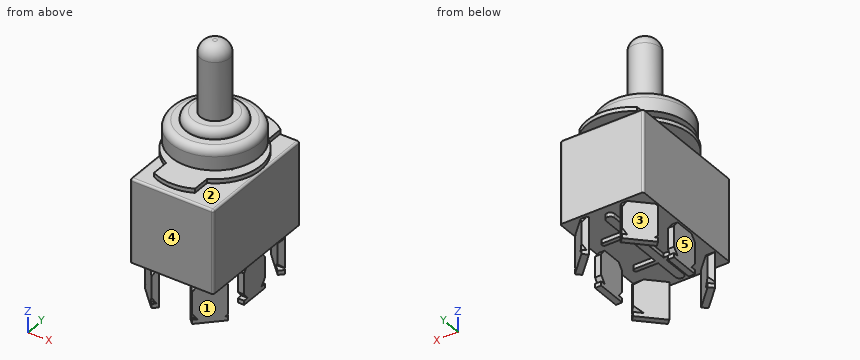
```python
from build123d import *

# Parameters (mm, degrees)
SKETCH_W     = 20
SKETCH_H     = 30
PAD_DEPTH    = 20
PAD001_DEPTH = 1.75
PAD002_DEPTH = 1
PAD003_DEPTH = 1.75
SKETCH004_R  = 10.5
PAD004_DEPTH = 5
SKETCH005_R  = 7
PAD005_DEPTH = 2
SKETCH006_R  = 3.5
PAD006_DEPTH = 17
FILLET_R     = 3
FILLET001_R  = 0.5
FILLET002_R  = 1.75
SKETCH007_W  = 1.5
SKETCH007_H  = 7.25
PAD007_DEPTH = 9
POCKET_DEPTH = 21.001
PAD008_DEPTH = 1


with BuildPart() as part:
    # Sketch → Pad (new body)
    with BuildSketch(Plane.XY):
        Rectangle(SKETCH_W, SKETCH_H)
    extrude(amount=PAD_DEPTH)

    # Sketch001 (on Face6 of Pad) → Pad001 (join)
    with BuildSketch(Plane.XY.offset(20)):
        Polygon((0, -8.313844), (7.2, -4.156922), (7.2, 4.156922), (0, 8.313844), (-7.2, 4.156922), (-7.2, -4.156922), align=None)
    extrude(amount=PAD001_DEPTH)

    # Sketch002 (on Face13 of Pad001) → Pad002 (join)
    with BuildSketch(Plane.XY.offset(21.75)):
        with BuildLine():
            ThreePointArc((6.924821, 12.746745), (0, 15.2), (-6.924821, 12.746745))
            Line((-6.924821, 8.546745), (-6.924821, 12.746745))
            ThreePointArc((-6.924821, 8.546745), (-10.934933, -1.194675), (-4.915971, -9.840388))
            Line((-4.915971, -9.840388), (-4.915971, -14.040388))
            ThreePointArc((-4.915971, -14.040388), (0, -15.2), (4.915971, -14.040388))
            Line((4.915971, -14.040388), (4.915971, -9.840388))
            ThreePointArc((4.915971, -9.840388), (10.934933, -1.194675), (6.924821, 8.546745))
            Line((6.924821, 12.746745), (6.924821, 8.546745))
        make_face()
    extrude(amount=PAD002_DEPTH)

    # Sketch003 (on Face22 of Pad002) → Pad003 (join)
    with BuildSketch(Plane.XY.offset(22.75)):
        Polygon((7.2, 4.156922), (0, 8.313844), (-7.2, 4.156922), (-7.2, -4.156922), (0, -8.313844), (7.2, -4.156922), align=None)
    extrude(amount=PAD003_DEPTH)

    # Sketch004 (on Face29 of Pad003) → Pad004 (join)
    with BuildSketch(Plane.XY.offset(24.5)):
        Circle(SKETCH004_R)
    extrude(amount=PAD004_DEPTH)

    # Sketch005 (on Face31 of Pad004) → Pad005 (join)
    with BuildSketch(Plane.XY.offset(29.5)):
        Circle(SKETCH005_R)
    extrude(amount=PAD005_DEPTH)

    # Sketch006 (on Face33 of Pad005) → Pad006 (join)
    with BuildSketch(Plane.XY.offset(31.5)):
        Circle(SKETCH006_R)
    extrude(amount=PAD006_DEPTH)

    # Fillet
    fillet_edges = [part.edges().sort_by_distance(p)[0] for p in [
        (-3.5, 0, 48.5),
    ]]
    fillet(fillet_edges, radius=FILLET_R)

    # Fillet001
    fillet001_edges = [part.edges().sort_by_distance(p)[0] for p in [
        (10, 15, 10),
        (10, -15, 10),
        (-10, -15, 10),
        (-10, 15, 10),
        (-10, 0, 20),
        (0, -15, 20),
        (10, 0, 20),
        (0, 15, 20),
    ]]
    fillet(fillet001_edges, radius=FILLET001_R)

    # Fillet002
    fillet002_edges = [part.edges().sort_by_distance(p)[0] for p in [
        (-10.5, 0, 29.5),
        (-7, 0, 31.5),
    ]]
    fillet(fillet002_edges, radius=FILLET002_R)

    # Sketch007 (on Face47 of Fillet002) → Pad007 (join)
    with BuildSketch(Plane(origin=(0, 0, 0), x_dir=(1, 0, 0), z_dir=(0, 0, -1))):
        Polygon((4.873476, 15), (10, 9.873476), (8.93934, 8.812816), (3.812816, 13.93934), align=None)
        with Locations((8.75, 0)):
            Rectangle(SKETCH007_W, SKETCH007_H)
        Polygon((-4.873476, 15), (-10, 9.873476), (-8.93934, 8.812816), (-3.812816, 13.93934), align=None)
        with Locations((-8.75, 0)):
            Rectangle(SKETCH007_W, SKETCH007_H)
        Polygon((4.873476, -15), (10, -9.873476), (8.93934, -8.812816), (3.812816, -13.93934), align=None)
        Polygon((-4.873476, -15), (-10, -9.873476), (-8.93934, -8.812816), (-3.812816, -13.93934), align=None)
    extrude(amount=PAD007_DEPTH)

    # Sketch008 (on Face39 of Pad007) → Pocket (cut, through all)
    with BuildSketch(Plane(origin=(-10, 0, 0), x_dir=(0, -1, 0), z_dir=(-1, 0, 0))):
        Polygon((-15, 0), (-15, -1.5), (-14.25, 0), align=None)
        Polygon((-8.812816, 0), (-8.812816, -1.5), (-10.312816, 0), align=None)
        Polygon((-15, -6.5), (-14.25, -8), (-15, -8), align=None)
        Polygon((-8.812816, -8), (-8.812816, -6.5), (-10.312816, -8), align=None)
        Polygon((15, 0), (15, -1.5), (14.25, 0), align=None)
        Polygon((8.812816, 0), (8.812816, -1.5), (10.312816, 0), align=None)
        Polygon((15, -6.5), (14.25, -8), (15, -8), align=None)
        Polygon((8.812816, -8), (8.812816, -6.5), (10.312816, -8), align=None)
        Polygon((-3.625, 0), (-3.625, -1.5), (-2.425, 0), align=None)
        Polygon((-3.625, -6.5), (-3.625, -8), (-2.425, -8), align=None)
        Polygon((3.625, 0), (3.625, -1.5), (2.425, 0), align=None)
        Polygon((3.625, -6.5), (3.625, -8), (2.425, -8), align=None)
    extrude(amount=-POCKET_DEPTH, mode=Mode.SUBTRACT)

    # Sketch009 (on Face50 of Pocket) → Pad008 (join)
    with BuildSketch(Plane(origin=(0, 0, 0), x_dir=(1, 0, 0), z_dir=(0, 0, -1))):
        with BuildLine():
            Line((-1, 12), (-1, 6))
            Line((-1, 6), (-6, 6))
            ThreePointArc((-6, 6), (-6.5, 5.5), (-6, 5))
            Line((-6, 5), (-1, 5))
            Line((-1, 5), (-1, -5))
            Line((-1, -5), (-6, -5))
            ThreePointArc((-6, -5), (-6.5, -5.5), (-6, -6))
            Line((-6, -6), (-1, -6))
            Line((-1, -6), (-1, -12))
            ThreePointArc((-1, -12), (-0.707107, -12.707107), (0, -13))
            ThreePointArc((0, -13), (0.707107, -12.707107), (1, -12))
            Line((1, -6), (1, -12))
            Line((6, -6), (1, -6))
            ThreePointArc((6, -6), (6.5, -5.5), (6, -5))
            Line((1, -5), (6, -5))
            Line((1, 5), (1, -5))
            Line((6, 5), (1, 5))
            ThreePointArc((6, 5), (6.5, 5.5), (6, 6))
            Line((1, 6), (6, 6))
            Line((1, 12), (1, 6))
            ThreePointArc((1, 12), (0.707107, 12.707107), (0, 13))
            ThreePointArc((0, 13), (-0.707107, 12.707107), (-1, 12))
        make_face()
    extrude(amount=PAD008_DEPTH)


solid = part.part
```
Work out the finished part from the listing and answer in its coordinate system (mm). Face numbers are marked on the shaded views. A direction names the side the tool comes from. Give positions to 0.01 mm unless a question says otherwise; leave off trailing zeros. Order: outer loops, then holes, each group sorted by start corner. A loop starts at its lowest first (then second) coordinate and runs counter-clockwise, first axis right, second up. Notation, with made-up numbers: (27, 32.25) - (33, 32.25) arc R29 cw to (33, 55.25) - close; hole circle Ø11 at (56, -11). An arc over 180 degrees is marked (long way). One line per item, written item: value. Start each with the question number.
1. Section C-C, the plane z = 37 is taken. Write down the section's boundary in (x, y), then the cut area to 3 significant figures.
2. Which of the six approach directions +Z, -Z, +X, -X, +Y, -Y give full straight-line access (tool end or side, diameter ignored) to the marked faces 3, 4 and 5?
3. Consider line 1 (Z direction, x = 3.5, y = 7); line 2 (X direction, y = -1, z = -6); line 3 (Z direction, x = -7.25, y = -6). Determine where each line is inside the solid, lowest interval first.
4. Section A-A, the plane z = 17 is taken. Write down the section's boundary in (x, y).
5. For a pull along Z with two mould halves and no side action, classify the marked faces 1 and 2 as released by +Z, released by -Z, zero draft, split by the parting line, or undercut.
6. Each of these flat-tipped pins is pushed along its axis until it touches: pin 1 Ø12 at (x, y) = (4.5, -6.5) entering from -Z; pin 2 Ø2 at (x, y) = (-4.5, 4.5) entering from +Z; pin 3 Ø1.1 at (x, z) = (-2.5, -0.5) entering from -Y; pin 4 Ø4 at (y, z) = (4, 9.5) entering from -X. Where does it stop, or does it pass through?
7. Section B-B, the plane z = 23.5 is taken. Write down the section's boundary in (x, y).
Filled sheet:
1. outline: circle Ø7 at (0, 0)
1. area: 38.5 mm²
2. face 3: -Z, -X, +Y
2. face 4: -Z, +X, -X, -Y
2. face 5: -Z, -X
3. line 1: 0 to 20, 21.75 to 22.75, 24.5 to 29.5
3. line 2: -9.5 to -8, 8 to 9.5
3. line 3: 0 to 20, 21.75 to 22.75, 24.5 to 29.37
4. outline: (-10, -14.5) arc R0.5 ccw to (-9.5, -15) - (9.5, -15) arc R0.5 ccw to (10, -14.5) - (10, 14.5) arc R0.5 ccw to (9.5, 15) - (-9.5, 15) arc R0.5 ccw to (-10, 14.5) - close
5. face 1: zero draft
5. face 2: undercut
6. pin 1: z = -9
6. pin 2: z = 31.5
6. pin 3: y = -15
6. pin 4: x = -10
7. outline: (-7.2, -4.16) - (0, -8.31) - (7.2, -4.16) - (7.2, 4.16) - (0, 8.31) - (-7.2, 4.16) - close
